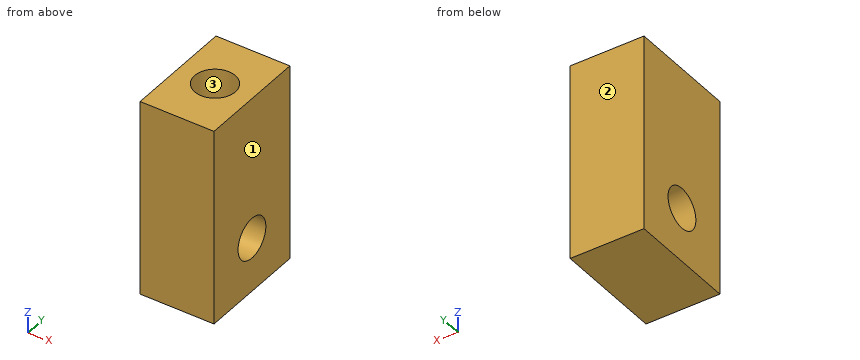
```python
from build123d import *

# Parameters (mm, degrees)
SKETCH1_W             = 6
SKETCH1_H             = 9
BOSS_EXTRUDE1_DEPTH   = 16
M4_TAPPED_HOLE1_D     = 3.3
M4_TAPPED_HOLE1_DEPTH = 6
M4_TAPPED_HOLE1_TIP   = 0.991420021
M4_TAPPED_HOLE2_D     = 3.3


with BuildPart() as part:
    # Sketch1 → Boss-Extrude1 (new body)
    with BuildSketch(Plane.XY):
        Rectangle(SKETCH1_W, SKETCH1_H)
    extrude(amount=BOSS_EXTRUDE1_DEPTH)

    # M4 Tapped Hole1
    with Locations(Plane.XY.offset(16)):
        with Locations((0, 0)):
            Hole(M4_TAPPED_HOLE1_D / 2, depth=M4_TAPPED_HOLE1_DEPTH)
            with Locations((0, 0, -(M4_TAPPED_HOLE1_DEPTH + M4_TAPPED_HOLE1_TIP / 2))):  # 118° drill point
                Cone(0, M4_TAPPED_HOLE1_D / 2, M4_TAPPED_HOLE1_TIP, mode=Mode.SUBTRACT)

    # M4 Tapped Hole2 (through all)
    with Locations(Plane(origin=(3, 0, 0), x_dir=(0, 0, -1), z_dir=(1, 0, 0))):
        with Locations((-4.411118023, 0)):
            Hole(M4_TAPPED_HOLE2_D / 2)


solid = part.part
```
Source: CAD feature listing. Evaluate the final solid. Frame: model axes, mm. Face numbers are marked on the shaded views. Coordinates: 2 decimals unless noted, no trailing zeros. Loops run counter-clockwise (first coordinate to the right, second up) from the corner with the lowest first, then second, coordinate; pieces in that order, holes last. Notation, with made-up numbers: M 85,37.5 L 120,37.5 A14 ccw 120,56.5 Z; hole C -27,42.5 d3. An arc over 180 degrees is marked long. Put each result on its own line as item: value. Start each with the question number.
1) Cut plane C-C on z = 3. Return the cut outline in (x, y).
2) Cut plane B-B on x = -1.9. Return the cut outline in (y, z), then the cut area to 3 significant figures.
3) Ray query, L1, parallel to Y at x = 0, z = 11.85; L2, parallel to X at y = 0, z = 13.6; L3, parallel to Y at x = 1.15, z = 15. Return the intervals inside material, ascending. Write a range as from..to.
4) Contact query for a flat-ended pin moving along its axis: pin 1 Ø3 at (x, y) = (0, 2) entering from -Z. Output: stop coordinate, or through.
5) Pull-direction query (Y, two-part tool) for the marked faces 1, 2 and 3; classes: pulls with the +Y half, pulls with the -Y half, needs draft (parallel to the pull), parting line crosses it, or undercut.
6) Cut plane A-A on z = 12.75. Return the cut outline in (x, y).
The answers:
1. outline: M -3,-4.5 L 3,-4.5 L 3,-0.86 L -3,-0.86 Z; M -3,0.86 L 3,0.86 L 3,4.5 L -3,4.5 Z
2. outline: M -4.5,0 L 4.5,0 L 4.5,16 L -4.5,16 Z; hole C 0,4.41 d3.3
2. area: 135 mm²
3. L1: y = -4.5..-1.65, 1.65..4.5
3. L2: x = -3..-1.65, 1.65..3
3. L3: y = -4.5..-1.18, 1.18..4.5
4. pin 1: stops at z = 0
5. face 1: needs draft
5. face 2: pulls with the +Y half
5. face 3: undercut
6. outline: M -3,-4.5 L 3,-4.5 L 3,4.5 L -3,4.5 Z; hole C 0,0 d3.3
